CAD build for the part. Positions are in the model's coordinates, mm. A direction names the side the tool comes from. Round coordinates to 2 decimals unless told otherwise and drop trailing zeros. Loops run counter-clockwise (first coordinate to the right, second up) from the corner with the lowest first, then second, coordinate; pieces in that order, holes last.
from build123d import *

# Parameters (mm, degrees)
SKETCH1_R           = 2
SKETCH1_R_2         = 1.5
BOSS_EXTRUDE1_DEPTH = 1.5


with BuildPart() as part:
    # Sketch1 → Boss-Extrude1 (new body, symmetric)
    with BuildSketch(Plane(origin=(0, 0, 0), x_dir=(1, 0, 0), z_dir=(0, 1, 0))):
        with BuildLine():
            Line((-10.519623347, 4), (-4.519623347, 4))
            ThreePointArc((-4.519623347, 4), (-3.055521732, 2.535898385), (-1.055521732, 2))
            Line((-1.055521732, 2), (15.834625342, 2))
            ThreePointArc((15.834625342, 2), (17.248838905, 2.258342613), (18.480376653, 3))
            Line((18.480376653, 3), (24.480376653, 3))
            ThreePointArc((24.480376653, 3), (27.480376653, 0), (24.480376653, -3))
            Line((24.480376653, -3), (18.480376653, -3))
            ThreePointArc((18.480376653, -3), (17.248838905, -2.258342613), (15.834625342, -2))
            Line((15.834625342, -2), (-1.055521732, -2))
            ThreePointArc((-1.055521732, -2), (-3.055521732, -2.535898385), (-4.519623347, -4))
            Line((-4.519623347, -4), (-10.519623347, -4))
            ThreePointArc((-10.519623347, -4), (-14.519623347, 0), (-10.519623347, 4))
        make_face()
        with Locations((-10.519623347, 0)):
            Circle(SKETCH1_R, mode=Mode.SUBTRACT)
        with Locations((24.480376653, 0)):
            Circle(SKETCH1_R_2, mode=Mode.SUBTRACT)
    extrude(amount=BOSS_EXTRUDE1_DEPTH, both=True)


solid = part.part
Item 1: Cut at C-C (x = 19.5). List the corners of the cut face in (y, z).
Verdict:
outline: (-1.5, -3) - (1.5, -3) - (1.5, 3) - (-1.5, 3) - close
Item 2: 3-axis set-ups, long thin cutter, end or side, ignore diameter. For faces 1 (the flat face through (21, 0, -3)), 2 (the cylindrical face through (17.268, 0.021, 2.266)), 3 (the flat face through (-8, 0, -4)), 4 (the flat face through (22, 0, 3)), 5 (the cylindrical face through (17.23, 0.02, -2.25)): which of +Z, -Z, +X, -X, +Y, -Y reach the whole face in a straight line?
Verdict:
face 1: -Z, +X, +Y, -Y
face 2: +Z, +Y, -Y
face 3: -Z, +X, -X, +Y, -Y
face 4: +Z, +X, +Y, -Y
face 5: -Z, +Y, -Y
Item 3: Cut at D-D (x = 12). List the corners of the cut face in (y, z).
Verdict:
outline: (-1.5, -2) - (1.5, -2) - (1.5, 2) - (-1.5, 2) - close
Item 4: Wall check: L1, parallel to X at y = 0.7, z = 0; L2, parallel to X at y = -1.3, z = 1.25; L3, parallel to Z at x = 10, y = -0.4. Give the ranges that are in metal, low to high.
Verdict:
L1: x = -14.52 to -12.52, -8.52 to 22.98, 25.98 to 27.48
L2: x = -14.32 to -12.08, -8.96 to 23.65, 25.31 to 27.21
L3: z = -2 to 2
Item 5: Cut at A-A (y = 0.7). List the corners of the cut face in (x, z).
Verdict:
outline: (-10.52, -4) - (-4.52, -4) arc R4 cw to (-1.06, -2) - (15.83, -2) arc R4 cw to (18.48, -3) - (24.48, -3) arc R3 ccw to (24.48, 3) - (18.48, 3) arc R4 cw to (15.83, 2) - (-1.06, 2) arc R4 cw to (-4.52, 4) - (-10.52, 4) arc R4 ccw to start; hole circle Ø4 at (-10.52, 0); hole circle Ø3 at (24.48, 0)
Item 6: Cut at B-B (z = 0). List the corners of the cut face in (x, y), plus the area to 3 significant figures.
Verdict:
outline: (-14.52, -1.5) - (-12.52, -1.5) - (-12.52, 1.5) - (-14.52, 1.5) - close; (-8.52, -1.5) - (22.98, -1.5) - (22.98, 1.5) - (-8.52, 1.5) - close; (25.98, -1.5) - (27.48, -1.5) - (27.48, 1.5) - (25.98, 1.5) - close
area: 105 mm2
Item 7: Mould opens along Z. For faces 6 (the flat face through (7, 0, -2)), 7 (the cylindrical face through (-3.03, 0.02, 2.52)), 8 (the cylindrical face through (-12.518, -0.021, -0.088)) say: released by +Z, released by -Z, zero draft, split by the parting line, or undercut.
Verdict:
face 6: released by -Z
face 7: released by +Z
face 8: undercut
Item 8: Flat gauge pins, fed straight in: P1, Ø1, axis at x = 19, y = 1, coming from the +Z side; P2, Ø1.5, axis at x = 22.5, y = -0.5, coming from the -Z side; P3, Ø4, axis at x = 24.48, z = 0, coming from the -Y side; P4, Ø1.5, axis at x = 6.5, y = 0, coming from the +Z side. Where does each tip first touch, or does it go through?
Verdict:
P1: stops at z = 3
P2: stops at z = -3
P3: stops at y = -1.5
P4: stops at z = 2
